Check sheet for the modelled part. Datum: model origin and axes. Units: mm. Round coordinates to 2 decimals unless told otherwise and drop trailing zeros. Loops run counter-clockwise (first coordinate to the right, second up) from the corner with the lowest first, then second, coordinate; pieces in that order, holes last. Notation, with made-up numbers: M -4.5,0.25 L 10.5,0.25 A30 cw 10.5,24.25 Z; hole C -11,30.5 d6. An arc over 180 degrees is marked long. One line per question, with ' | ' between items. Start each with the question number.
(1) Section check A-A (z = 3.75). Record the boundary of the cut face in (x, y), and give its area (3 significant figures).
(2) Go/stop test with flat-tipped pins: P1, Ø2, axis at y = 46.5, z = 4.5, coming from the +X side; P2, Ø2.5, axis at x = -54, y = 47.5, coming from the +Z side. Record where each tip stops, or that it passes through.
(3) Thickness scan on probe 1 along X at (y, z) = (47.1, 0.5); probe 2 along Y at (x, z) = (-51.7, -4.5); probe 3 along Z at (x, y) = (-52.45, 46.9). Record the ranges inside material, lowest first. Write a range as [from, to].
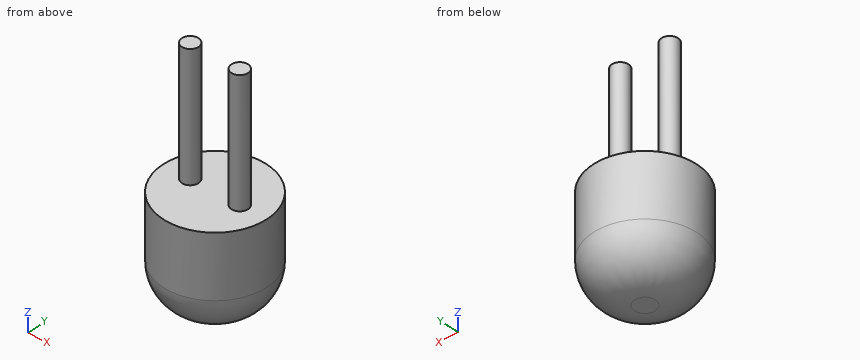
```python
from build123d import *

# Parameters (mm, degrees)
SKETCH1_R           = 2.5
BOSS_EXTRUDE1_DEPTH = 5
SKETCH2_R           = 0.4
BOSS_EXTRUDE2_DEPTH = 6
FILLET1_R           = 2


with BuildPart() as part:
    # Sketch1 → Boss-Extrude1 (new body)
    with BuildSketch(Plane.XY):
        with Locations((-53, 47)):
            Circle(SKETCH1_R)
    extrude(amount=-BOSS_EXTRUDE1_DEPTH)

    # Sketch2 → Boss-Extrude2 (add)
    with BuildSketch(Plane.XY):
        with Locations((-54.191552133, 47)):
            Circle(SKETCH2_R)
        with Locations((-51.808447867, 47)):
            Circle(SKETCH2_R)
    extrude(amount=BOSS_EXTRUDE2_DEPTH)

    # Fillet1
    fillet1_edges = [part.edges().sort_by_distance(p)[0] for p in [
        (-55.5, 47, -5),
    ]]
    fillet(fillet1_edges, radius=FILLET1_R)


solid = part.part
```
The answers:
1) outline: C -54.19,47 d0.8; C -51.81,47 d0.8 | area: 1.01 mm²
2) P1: x = -51.41 | P2: z = 6
3) probe 1: [-54.58, -53.8], [-52.2, -51.42] | probe 2: [45.72, 48.28] | probe 3: [-5, 0]
